from build123d import *

# Parameters (mm, degrees)
BOSS_EXTRUDE1_DEPTH = 6.35
SKETCH2_R           = 1.651
CUT_EXTRUDE1_DEPTH  = 23.368
SKETCH3_R           = 1.651
CUT_EXTRUDE2_DEPTH  = 23.368
SKETCH4_R           = 1.651
CUT_EXTRUDE3_DEPTH  = 23.368
SKETCH5_R           = 1.651
CUT_EXTRUDE4_DEPTH  = 23.368
SKETCH6_R           = 6.35
CUT_EXTRUDE5_DEPTH  = 14.3002


with BuildPart() as part:
    # Sketch1 → Boss-Extrude1 (new body)
    with BuildSketch(Plane(origin=(0, 0, 0), x_dir=(1, 0, 0), z_dir=(0, 1, 0))):
        with BuildLine():
            Line((-3.175, 18.783553311), (-3.175, 28.943553311))
            Line((-3.175, 28.943553311), (-10.16, 28.943553311))
            Line((-10.16, 28.943553311), (-10.16, 16.114493476))
            ThreePointArc((-10.16, 16.114493476), (-13.470384182, 13.470384182), (-16.114493476, 10.16))
            Line((-16.114493476, 10.16), (-28.943553311, 10.16))
            Line((-28.943553311, 10.16), (-28.943553311, 3.175))
            Line((-28.943553311, 3.175), (-18.783553311, 3.175))
            ThreePointArc((-18.783553311, 3.175), (-19.05, 0), (-18.783553311, -3.175))
            Line((-18.783553311, -3.175), (-28.943553311, -3.175))
            Line((-28.943553311, -3.175), (-28.943553311, -10.16))
            Line((-28.943553311, -10.16), (-16.114493476, -10.16))
            ThreePointArc((-16.114493476, -10.16), (-13.470384182, -13.470384182), (-10.16, -16.114493476))
            Line((-10.16, -16.114493476), (-10.16, -28.943553311))
            Line((-10.16, -28.943553311), (-3.175, -28.943553311))
            Line((-3.175, -28.943553311), (-3.175, -18.783553311))
            ThreePointArc((-3.175, -18.783553311), (0, -19.05), (3.175, -18.783553311))
            Line((3.175, -18.783553311), (3.175, -28.943553311))
            Line((3.175, -28.943553311), (10.144252899, -28.943553311))
            Line((10.144252899, -28.943553311), (10.144252899, -16.124411094))
            ThreePointArc((10.144252899, -16.124411094), (13.463802963, -13.476962186), (16.114493476, -10.16))
            Line((16.114493476, -10.16), (28.943553311, -10.16))
            Line((28.943553311, -10.16), (28.943553311, -3.175))
            Line((28.943553311, -3.175), (18.783553311, -3.175))
            ThreePointArc((18.783553311, -3.175), (19.05, 0), (18.783553311, 3.175))
            Line((18.783553311, 3.175), (28.943553311, 3.175))
            Line((28.943553311, 3.175), (28.943553311, 10.146623982))
            Line((28.943553311, 10.146623982), (16.122919145, 10.146623982))
            ThreePointArc((16.122919145, 10.146623982), (13.475972183, 13.464793861), (10.16, 16.114493476))
            Line((10.16, 16.114493476), (10.16, 28.943553311))
            Line((10.16, 28.943553311), (3.175, 28.943553311))
            Line((3.175, 28.943553311), (3.175, 18.783553311))
            ThreePointArc((3.175, 18.783553311), (0, 19.05), (-3.175, 18.783553311))
        make_face()
    extrude(amount=BOSS_EXTRUDE1_DEPTH)

    # Sketch2 → Cut-Extrude1 (cut)
    with BuildSketch(Plane(origin=(10.16, 0, 0), x_dir=(0, 0, -1), z_dir=(1, 0, 0))):
        with Locations((25.768553311, 3.175)):
            Circle(SKETCH2_R)
    extrude(amount=-CUT_EXTRUDE1_DEPTH, mode=Mode.SUBTRACT)

    # Sketch3 → Cut-Extrude2 (cut)
    with BuildSketch(Plane(origin=(0, 0, -10.146623982), x_dir=(-1, 0, 0), z_dir=(0, 0, -1))):
        with Locations((-25.768553311, 3.175)):
            Circle(SKETCH3_R)
    extrude(amount=-CUT_EXTRUDE2_DEPTH, mode=Mode.SUBTRACT)

    # Sketch4 → Cut-Extrude3 (cut)
    with BuildSketch(Plane(origin=(10.144252899, 0, 0), x_dir=(0, 0, -1), z_dir=(1, 0, 0))):
        with Locations((-25.768553311, 3.175)):
            Circle(SKETCH4_R)
    extrude(amount=-CUT_EXTRUDE3_DEPTH, mode=Mode.SUBTRACT)

    # Sketch5 → Cut-Extrude4 (cut)
    with BuildSketch(Plane.XY.offset(10.16)):
        with Locations((-25.768553311, 3.175)):
            Circle(SKETCH5_R)
    extrude(amount=-CUT_EXTRUDE4_DEPTH, mode=Mode.SUBTRACT)

    # Sketch6 → Cut-Extrude5 (cut)
    with BuildSketch(Plane(origin=(0, 6.35, 0), x_dir=(1, 0, 0), z_dir=(0, 1, 0))):
        with Locations(Location((0, 0, 0), (0, 0, 270))):
            Circle(SKETCH6_R)
    extrude(amount=-CUT_EXTRUDE5_DEPTH, mode=Mode.SUBTRACT)


solid = part.part
Design review of the part built by this model. Coordinates are the model's own, in mm. A direction names the side the tool comes from. Give positions to 0.01 mm unless a question says otherwise; leave off trailing zeros. Loops run counter-clockwise (first coordinate to the right, second up) from the corner with the lowest first, then second, coordinate; pieces in that order, holes last. Notation, with made-up numbers: (28, 27.25) - (43, 27.25) arc R20 ccw to (43, 62.25) - close; hole circle Ø1 at (71, -21). An arc over 180 degrees is marked (long way). Write item = value, one per line.
1) To check wall thickness, follow line 1 (X direction, y = 4.5, z = 24.5) (3 decimals); line 2 (Z direction, x = 21, y = 1.25) (3 decimals); line 3 (Z direction, x = -5, y = 1.75). State the ranges of each line that lie inside material, in increasing order.
Result sheet:
line_1 = -10.16 to -3.175, 3.175 to 10.144
line_2 = -10.147 to -3.175, 3.175 to 10.16
line_3 = -28.94 to -26.6, -24.93 to -3.91, 3.91 to 24.93, 26.6 to 28.94
2) Draft analysis for pull direction Z (two halves, no side actions). For faces 6 (the face through (3.175, 3.1, 23.8)), 7 (the face through (19.05, 3.13, 0.04)), 8 (the face through (7, 3, -28.944)), state which applies: +Z half, -Z half, draft (parallel to the pull), parting line (faces both ways), or undercut.
Result sheet:
face_6 = draft
face_7 = undercut
face_8 = -Z half
3) Take a section at A-A on z = 0. State the section outline as (x, y) points.
Result sheet:
outline = (-19.05, 0) - (-6.35, 0) - (-6.35, 6.35) - (-19.05, 6.35) - close; (6.35, 0) - (19.05, 0) - (19.05, 6.35) - (6.35, 6.35) - close
4) Take a section at D-D on z = 7.5. State the section outline as (x, y) points (3 decimals), and give its area (3 significant figures).
Result sheet:
outline = (-28.944, 0) - (28.944, 0) - (28.944, 6.35) - (-28.944, 6.35) - close; hole circle Ø3.302 at (-25.769, 3.175); hole circle Ø3.302 at (25.769, 3.175)
area = 350 mm2
5) Tool access review of faces 1 (the face through (-10.16, 3, 22)), 2 (the face through (-3.175, 3.1, -23.8)), 3 (the face through (23.9, 3.1, 3.175)), 4 (the face through (-10.16, 3, -23)), 5 (the face through (23, 3, -10.147)): name each direction out of +Z, -Z, +X, -X, +Y, -Y from which nothing blocks a thin tool from reaching the whole face with its end or side.
Result sheet:
face_1 = +Z, -X, +Y, -Y
face_2 = -Z, +Y, -Y
face_3 = +X, +Y, -Y
face_4 = -Z, -X, +Y, -Y
face_5 = -Z, +X, +Y, -Y
6) Clearance check with flat-ended pins moving along their axes: pin 1 Ø1.9 at (y, z) = (4, 22.5) entering from -X; pin 2 Ø6 at (x, z) = (-3.5, -14) entering from -Y; pin 3 Ø1 at (x, y) = (-20.5, 2) entering from -Z; pin 4 Ø2 at (y, z) = (1, 21.5) entering from +X. State where each tip first meets the part, or that it passes through.
Result sheet:
pin_1 = -10.16
pin_2 = 0
pin_3 = -10.16
pin_4 = 10.14
7) Take a section at B-B on x = 22. State the section outline as (y, z) points (3 decimals).
Result sheet:
outline = (0, -10.147) - (6.35, -10.147) - (6.35, -3.175) - (0, -3.175) - close; (0, 3.175) - (6.35, 3.175) - (6.35, 10.16) - (0, 10.16) - close
